Could you check a few things on this model? Use its own coordinates, in mm. A direction names the side the tool comes from. Round coordinates to 2 decimals unless told otherwise and drop trailing zeros. Loops run counter-clockwise (first coordinate to the right, second up) from the corner with the lowest first, then second, coordinate; pieces in that order, holes last. Notation, with made-up numbers: (19.5, 68) - (67.5, 68) arc R18 cw to (67.5, 90) - close; hole circle Ø3 at (38, 59). An arc over 180 degrees is marked (long way). Answer as CSV lines item,"result". Start each with the question number.
1) Suppose I cut it at D-D, the plane z = 25. Write out the boundary of the cut face in (x, y).
2) Suppose I cut it at A-A, the plane y = 60. Write out the boundary of the cut face in (x, z), then the cut area to 3 significant figures.
3) Suppose I cut it at B-B, the plane x = -40. Write out the boundary of the cut face in (y, z).
4) Please list where these lines run through material, in increasing order: line 1 along Y through (x, z) = (39.75, 25); line 2 along Z through (x, y) = (-18, 97); line 3 along Y through (x, z) = (1.5, 7).
5) I'm going to push flat-ended pins straight in: pin 1 Ø3 at (y, z) = (113, 45) entering from -X; pin 2 Ø6 at (y, z) = (85.5, 20.5) entering from +X; pin 3 Ø1 at (x, z) = (10.5, 20.5) entering from -Y. Where does each tip first touch, or does it pass through?
6) Suppose I cut it at C-C, the plane z = 5. Write out the boundary of the cut face in (x, y).
7) Which directions (+Z, -Z, +X, -X, +Y, -Y) give clear straight access to the entire face, cutting with the end or side of a thin tool? Please do faces 1 (the face through (30, 110, 25)), 2 (the face through (0, 5, 5)), 3 (the face through (0, 115, 5)), 4 (the face through (55, 30, 25)).
8) We'd pull the mould along Y, two halves only. Please class faces 5 (the face through (10, 25, 25)), 6 (the face through (20, 100, 25)), 7 (the face through (20, 20, 25)), 8 (the face through (55, 90, 25)): pulls with the +Y half, pulls with the -Y half, needs draft (parallel to the pull), parting line crosses it, or undercut.
```python
from build123d import *

# Parameters (mm, degrees)
BOSS_EXTRUDE1_DEPTH = 50
SKETCH2_W           = 10
SKETCH2_H           = 60
CUT_EXTRUDE1_DEPTH  = 50
CUT_EXTRUDE2_DEPTH  = 50
SKETCH4_W           = 60
SKETCH4_H           = 30
CUT_EXTRUDE3_DEPTH  = 177
SKETCH5_R           = 16
CUT_EXTRUDE5_DEPTH  = 177
SKETCH6_W           = 20
SKETCH6_H           = 30
CUT_EXTRUDE6_DEPTH  = 20
SKETCH7_W           = 20
SKETCH7_H           = 30
CUT_EXTRUDE7_DEPTH  = 20


with BuildPart() as part:
    # Sketch1 → Boss-Extrude1 (new body)
    with BuildSketch(Plane.XY):
        with BuildLine():
            Line((0, 120), (0, 110))
            ThreePointArc((0, 110), (-50, 60), (0, 10))
            Line((0, 10), (0, 0))
            Line((0, 0), (60, 0))
            Line((60, 0), (60, 120))
            Line((60, 120), (0, 120))
        make_face()
    extrude(amount=BOSS_EXTRUDE1_DEPTH)

    # Sketch2 → Cut-Extrude1 (cut)
    with BuildSketch(Plane.XY.offset(50)):
        with Locations((55, 60)):
            Rectangle(SKETCH2_W, SKETCH2_H)
    extrude(amount=-CUT_EXTRUDE1_DEPTH, mode=Mode.SUBTRACT)

    # Sketch3 → Cut-Extrude2 (cut)
    with BuildSketch(Plane.XY.offset(50)):
        with BuildLine():
            Line((30, 90), (30, 30))
            Line((30, 30), (0, 30))
            ThreePointArc((0, 30), (-30, 60), (0, 90))
            Line((0, 90), (30, 90))
        make_face()
    extrude(amount=-CUT_EXTRUDE2_DEPTH, mode=Mode.SUBTRACT)

    # Sketch4 → Cut-Extrude3 (cut)
    with BuildSketch(Plane(origin=(0, 120, 0), x_dir=(1, 0, 0), z_dir=(0, 1, 0))):
        with Locations((-20, -25)):
            Rectangle(SKETCH4_W, SKETCH4_H)
    extrude(amount=-CUT_EXTRUDE3_DEPTH, mode=Mode.SUBTRACT)

    # Sketch5 → Cut-Extrude5 (cut)
    with BuildSketch(Plane.ZY.offset(-30)):
        with Locations((25, 60)):
            Circle(SKETCH5_R)
    extrude(amount=-CUT_EXTRUDE5_DEPTH, mode=Mode.SUBTRACT)

    # Sketch6 → Cut-Extrude6 (cut)
    with BuildSketch(Plane(origin=(0, 120, 0), x_dir=(1, 0, 0), z_dir=(0, 1, 0))):
        with Locations((20, -25)):
            Rectangle(SKETCH6_W, SKETCH6_H)
    extrude(amount=-CUT_EXTRUDE6_DEPTH, mode=Mode.SUBTRACT)

    # Sketch7 → Cut-Extrude7 (cut)
    with BuildSketch(Plane.XZ):
        with Locations((20, 25)):
            Rectangle(SKETCH7_W, SKETCH7_H)
    extrude(amount=-CUT_EXTRUDE7_DEPTH, mode=Mode.SUBTRACT)


solid = part.part
```
Filled sheet:
1,outline,"(10, 20) - (30, 20) - (30, 0) - (60, 0) - (60, 30) - (50, 30) - (50, 44) - (30, 44) - (30, 30) - (10, 30) - close; (10, 90) - (30, 90) - (30, 76) - (50, 76) - (50, 90) - (60, 90) - (60, 120) - (30, 120) - (30, 100) - (10, 100) - close"
2,outline,"(-50, 0) - (-30, 0) - (-30, 10) - (-50, 10) - close; (-50, 40) - (-30, 40) - (-30, 50) - (-50, 50) - close; (30, 0) - (50, 0) - (50, 9) - (30, 9) - close; (30, 41) - (50, 41) - (50, 50) - (30, 50) - close"
2,area,"760 mm²"
3,outline,"(30, 0) - (90, 0) - (90, 10) - (30, 10) - close; (30, 40) - (90, 40) - (90, 50) - (30, 50) - close"
4,line 1,"0 to 44, 76 to 120"
4,line 2,"0 to 10, 40 to 50"
4,line 3,"0 to 30, 90 to 120"
5,pin 1,"x = 0"
5,pin 2,"x = 50"
5,pin 3,"y = 20"
6,outline,"(0, 0) - (60, 0) - (60, 30) - (50, 30) - (50, 90) - (60, 90) - (60, 120) - (0, 120) - (0, 110) arc R50 ccw to (0, 10) - close; hole (0, 30) - (30, 30) - (30, 90) - (0, 90) arc R30 ccw to start"
7,face 1,"-X, +Y"
7,face 2,"+Z, -Z, -X, -Y"
7,face 3,"+Z, -Z, -X, +Y"
7,face 4,"+Z, -Z, +X"
8,face 5,"needs draft"
8,face 6,"pulls with the +Y half"
8,face 7,"pulls with the -Y half"
8,face 8,"undercut"
